Autodesk Inventor part; units mm, degrees
ref_plane "YZ Plane" through (0, 0, 0) normal (1, 0, 0) x (0, 1, 0)
ref_plane "XZ Plane" through (0, 0, 0) normal (0, 1, 0) x (-1, 0, 0)
ref_plane "XY Plane" through (0, 0, 0) normal (0, 0, 1) x (1, 0, 0)
sketch "Sketch1" plane through (0, 0, 0) normal (0, 1, 0) x (-1, 0, 0)
  line L0 (0, 4.0415) -> (3.5, 2.0207)
  line L1 (3.5, 2.0207) -> (3.5, -2.0207)
  line L2 (3.5, -2.0207) -> (0, -4.0415)
  line L3 (0, -4.0415) -> (-3.5, -2.0207)
  line L4 (-3.5, -2.0207) -> (-3.5, 2.0207)
  line L5 (-3.5, 2.0207) -> (0, 4.0415)
  point P0 (0, 0)
  point P1 (0, 0)
  dimension "d0" = 3.5
extrude "Extrusion1" add sketch "Sketch1" along normal blind 3.2
sketch "Sketch2" plane through (0, 3.2, 0) normal (0, 1, 0) x (1, 0, 0)
  circle A0 centre (0, 0) radius 2
  dimension "d3" = 4
extrude "Extrusion2" cut sketch "Sketch2" against normal blind 4.3
thread "Thread1"
properties part number "M4Nut" material "Steel, Alloy"
Input: part model. Units: mm. Frame: model coordinates. Give positions to 0.01 mm unless a question says otherwise; leave off trailing zeros. Loops run counter-clockwise (first coordinate to the right, second up) from the corner with the lowest first, then second, coordinate; pieces in that order, holes last. Notation, with made-up numbers: (11.25, -23.5) -> (55.25, -23.5) arc R21 cw to (55.25, -19.5) -> close; hole circle Ø7 at (31.5, -26). An arc over 180 degrees is marked (long way). Use a Markdown table: item, result.
Q1. Section query D-D, the plane x = -2.75. Return the cut outline in (y, z), plus the area to 3 significant figures.
Entries:
| item | result |
|---|---|
| outline | (0, -2.45) -> (3.2, -2.45) -> (3.2, 2.45) -> (0, 2.45) -> close |
| area | 15.7 mm² |
Q2. First-contact query: P1, Ø1, axis at x = 1, y = 2.5, coming from the -Z side. Flat tip, straight axial feed; report the tip coordinate or a pass-through.
Entries:
| item | result |
|---|---|
| P1 | stops at z = -3.75 |
Q3. Section query A-A, the plane y = 0.25. Return the cut outline in (x, z), plus the area to 3 significant figures.
Entries:
| item | result |
|---|---|
| outline | (-3.5, -2.02) -> (0, -4.04) -> (3.5, -2.02) -> (3.5, 2.02) -> (0, 4.04) -> (-3.5, 2.02) -> close; hole circle Ø4 at (0, 0) |
| area | 29.9 mm² |
Q4. Section query C-C, the plane x = -0.25. Return the cut outline in (y, z), plus the area to 3 significant figures.
Entries:
| item | result |
|---|---|
| outline | (0, -3.9) -> (3.2, -3.9) -> (3.2, -1.98) -> (0, -1.98) -> close; (0, 1.98) -> (3.2, 1.98) -> (3.2, 3.9) -> (0, 3.9) -> close |
| area | 12.2 mm² |
Q5. Section query B-B, the plane z = 0. Return the cut outline in (x, y), plus the area to 3 significant figures.
Entries:
| item | result |
|---|---|
| outline | (-3.5, 0) -> (-2, 0) -> (-2, 3.2) -> (-3.5, 3.2) -> close; (2, 0) -> (3.5, 0) -> (3.5, 3.2) -> (2, 3.2) -> close |
| area | 9.60 mm² |
Q6. Ray query, probe 1 along X at (y, z) = (0.25, 1.75); probe 2 along X at (y, z) = (2.05, 0); probe 3 along Z at (x, y) = (-1, 1.65). Return the intervals inside material, ascending. Write a range as from..to.
Entries:
| item | result |
|---|---|
| probe 1 | x = -3.5..-0.97, 0.97..3.5 |
| probe 2 | x = -3.5..-2, 2..3.5 |
| probe 3 | z = -3.46..-1.73, 1.73..3.46 |
Q7. Pull-direction query (X, two-part tool) for faces 1 (the flat face through (2, 3.2, -2)), 2 (the cylindrical face through (0, 2, 2)), 3 (the flat face through (3.5, 2, 0)); classes: pulls with the +X half, pulls with the -X half, needs draft (parallel to the pull), parting line crosses it, or undercut.
Entries:
| item | result |
|---|---|
| face 1 | needs draft |
| face 2 | undercut |
| face 3 | pulls with the +X half |
